from build123d import *

# Parameters (mm, degrees)
SKETCH1_R           = 1
BOSS_EXTRUDE2_DEPTH = 2.5
SKETCH2_R           = 1
SKETCH2_W           = 20
SKETCH2_H           = 3
CUT_EXTRUDE1_DEPTH  = 28.041634566


with BuildPart() as part:
    # Sketch1 → Boss-Extrude2 (new, symmetric)
    with BuildSketch(Plane.XY):
        with BuildLine():
            Line((7.5, 15), (15, 15))
            ThreePointArc((15, 15), (17.5, 17.5), (15, 20))
            Line((15, 20), (-15, 20))
            ThreePointArc((-15, 20), (-17.5, 17.5), (-15, 15))
            Line((-15, 15), (-7.5, 15))
            Line((-7.5, 15), (-7.5, -15))
            Line((-7.5, -15), (-15, -15))
            ThreePointArc((-15, -15), (-17.5, -17.5), (-15, -20))
            Line((-15, -20), (15, -20))
            ThreePointArc((15, -20), (17.5, -17.5), (15, -15))
            Line((15, -15), (7.5, -15))
            Line((7.5, -15), (7.5, 15))
        make_face()
        with Locations((-15, 17.5)):
            Circle(SKETCH1_R, mode=Mode.SUBTRACT)
        with Locations((15, 17.5)):
            Circle(SKETCH1_R, mode=Mode.SUBTRACT)
        with Locations(Location((15, -17.5, 0), (0, 0, 180))):
            Circle(SKETCH1_R, mode=Mode.SUBTRACT)
        with Locations(Location((-15, -17.5, 0), (0, 0, 180))):
            Circle(SKETCH1_R, mode=Mode.SUBTRACT)
    extrude(amount=BOSS_EXTRUDE2_DEPTH, both=True)

    # Sketch2 → Cut-Extrude1 (cut, through all)
    with BuildSketch(Plane.XY.offset(2.5)):
        Circle(SKETCH2_R)
        with Locations((0, 17.5)):
            Rectangle(SKETCH2_W, SKETCH2_H)
        with Locations((0, -17.5)):
            Rectangle(SKETCH2_W, SKETCH2_H)
    extrude(amount=-CUT_EXTRUDE1_DEPTH, mode=Mode.SUBTRACT)


solid = part.part
Could you check a few things on this model? Use its own coordinates, in mm. A direction names the side the tool comes from. Round coordinates to 2 decimals unless told otherwise and drop trailing zeros. Write each loop counter-clockwise with the first axis right and the second up, starting at its lowest first coordinate (ties: lowest second). Pieces come first, ordered by that corner, then holes. Notation, with made-up numbers: (17.5, 16) -> (33.5, 16) arc R25 cw to (33.5, 45) -> close; hole circle Ø6 at (17, 87.25). An arc over 180 degrees is marked (long way). Use a Markdown table: item, result.
1. If we section it at D-D (y = -17.5): List the corners of the cut face in (x, z) for me, then the cut area to 3 significant figures.
Answer key:
| item | result |
|---|---|
| outline | (-17.5, -2.5) -> (-16, -2.5) -> (-16, 2.5) -> (-17.5, 2.5) -> close; (-14, -2.5) -> (-10, -2.5) -> (-10, 2.5) -> (-14, 2.5) -> close; (10, -2.5) -> (14, -2.5) -> (14, 2.5) -> (10, 2.5) -> close; (16, -2.5) -> (17.5, -2.5) -> (17.5, 2.5) -> (16, 2.5) -> close |
| area | 55.0 mm^2 |
2. If we section it at B-B (y = 0): List the corners of the cut face in (x, z) for me, then the cut area to 3 significant figures.
Answer key:
| item | result |
|---|---|
| outline | (-7.5, -2.5) -> (-1, -2.5) -> (-1, 2.5) -> (-7.5, 2.5) -> close; (1, -2.5) -> (7.5, -2.5) -> (7.5, 2.5) -> (1, 2.5) -> close |
| area | 65.0 mm^2 |
3. Which directions (+Z, -Z, +X, -X, +Y, -Y) give clear straight access to the entire face, cutting with the end or side of a thin tool? Please do faces 1 (the face through (-1, -1, -2.5)), 2 (the face through (11, 15, 0)), 3 (the face through (10, -18, 0)).
Answer key:
| item | result |
|---|---|
| face 1 | -Z, +X, -X, +Y, -Y |
| face 2 | +Z, -Z, +X |
| face 3 | +Z, -Z |
4. For pin 1 Ø1.5 at (y, z) = (3, -1) entering from -X, with a flat end and sliding along its axis, tell me the tip position at first contact or that it passes through.
Answer key:
| item | result |
|---|---|
| pin 1 | stops at x = -7.5 |
5. Please list where these lines run through material, in increasing order: probe 1 along X at (y, z) = (-17.5, 1.1); probe 2 along Y at (x, z) = (-15, -1); probe 3 along Y at (x, z) = (-4, 1.9).
Answer key:
| item | result |
|---|---|
| probe 1 | x = -17.5 to -16, -14 to -10, 10 to 14, 16 to 17.5 |
| probe 2 | y = -20 to -18.5, -16.5 to -15, 15 to 16.5, 18.5 to 20 |
| probe 3 | y = -20 to -19, -16 to 16, 19 to 20 |
6. We'd pull the mould along X, two halves only. Please class faces 4 (the face through (-14.54, 16.61, -0.04)), 5 (the face through (17.5, 17.4, 0)), 6 (the face through (-17.5, -17.4, 0)), 7 (the face through (-1, -1, 2.5)): +X half, -X half, draft (parallel to the pull), parting line (faces both ways), or undercut.
Answer key:
| item | result |
|---|---|
| face 4 | undercut |
| face 5 | +X half |
| face 6 | -X half |
| face 7 | draft |
7. If we section it at C-C (x = 13): List the corners of the cut face in (y, z) for me, then the cut area to 3 significant figures.
Answer key:
| item | result |
|---|---|
| outline | (-20, -2.5) -> (-15, -2.5) -> (-15, 2.5) -> (-20, 2.5) -> close; (15, -2.5) -> (20, -2.5) -> (20, 2.5) -> (15, 2.5) -> close |
| area | 50.0 mm^2 |
8. If we section it at A-A (x = -6.5): List the corners of the cut face in (y, z) for me, then the cut area to 3 significant figures.
Answer key:
| item | result |
|---|---|
| outline | (-20, -2.5) -> (-19, -2.5) -> (-19, 2.5) -> (-20, 2.5) -> close; (-16, -2.5) -> (16, -2.5) -> (16, 2.5) -> (-16, 2.5) -> close; (19, -2.5) -> (20, -2.5) -> (20, 2.5) -> (19, 2.5) -> close |
| area | 170 mm^2 |
